Geometry: final body of the model. Coordinates: model frame, mm. A direction names the side the tool comes from. Give positions to 0.01 mm unless a question says otherwise; leave off trailing zeros. Write each loop counter-clockwise with the first axis right and the second up, starting at its lowest first coordinate (ties: lowest second). Pieces come first, ordered by that corner, then holes. Notation, with made-up numbers: M 40,32.5 L 47,32.5 A12 cw 47,48.5 Z; hole C 77,57 d8. An arc over 180 degrees is marked long. Use one line per item in the form item = value. Start each with the question number.
Item 1: Section query B-B on x = -7.5. Return loops of the section in (y, z) (3 decimals), then the cut area to 4 significant figures.
Item 2: Access query for faces 1 (the flat face through (27, 2, 5)), 2 (the flat face through (-27, 2, 15)), 3 (the flat face through (-25.85, 2, -18)). Directions: +Z, -Z, +X, -X, +Y, -Y. A direction counts if a zero-diameter tool reaches every point of the face in a straight line with its end or side. Return the directions, or none.
Item 3: Section query A-A on z = 17. Return loops of the section in (x, y) (3 decimals).
Item 4: Section query C-C on y = 2.4. Give the number of separate pieces and of enclosed holes in the cut face, then the cut area to 3 significant figures.
Item 5: Material intervals for line 1 along Z through (x, y) = (3, 1.9) (3 decimals); line 2 along X through (y, z) = (3.2, 1) (3 decimals); line 3 along X through (y, z) = (1, 24.3) (3 decimals), sorted ascending. Write a range as from..to.
Item 6: Section query D-D on z = -24.3. Return loops of the section in (x, y) (3 decimals), then the cut area to 3 significant figures.
Item 7: Contact query for flat-ended pins moving along their axis: P1, Ø1.5, axis at x = 27.5, y = 2.5, coming from the +Z side; P2, Ø2.5, axis at y = 1.5, z = 18.5, coming from the +X side; P3, Ø1, axis at x = 23, y = 2, coming from the +Z side. Output: stop coordinate, or through.
Item 8: Pull-direction query (X, two-part tool) for faces 4 (the flat face through (28.85, 2, 10)), 5 (the flat face through (-12, 5, 0)), 6 (the cylindrical face through (4.205, 2.465, -22.683)); classes: released by +X, released by -X, zero draft, split by the parting line, or undercut.
from build123d import *

# Parameters (mm, degrees)
SKETCH_1_R      = 1.75
SKETCH_1_W      = 20.75
SKETCH_1_H      = 41.25
EXTRUDE_1_DEPTH = 5
FILLET_1_R      = 8


with BuildPart() as part:
    # 草图1 → 凸台-拉伸1 (new body)
    with BuildSketch(Plane(origin=(0, 0, 0), x_dir=(1, 0, 0), z_dir=(0, 1, 0))):
        Polygon((25.85, -30), (-25.85, -30), (-25.85, -15), (-28.85, -15), (-28.85, -5), (-25.85, -5), (-25.85, 5), (-28.85, 5), (-28.85, 15), (-25.85, 15), (-25.85, 30), (25.85, 30), (25.85, 15), (28.85, 15), (28.85, 5), (25.85, 5), (25.85, -5), (28.85, -5), (28.85, -15), (25.85, -15), align=None)
        with Locations(Location((-4.875, -24.3, 0), (0, 0, 270))):
            Circle(SKETCH_1_R, mode=Mode.SUBTRACT)
        with Locations(Location((4.875, -24.3, 0), (0, 0, 90))):
            Circle(SKETCH_1_R, mode=Mode.SUBTRACT)
        with Locations(Location((4.875, 24.3, 0), (0, 0, 270))):
            Circle(SKETCH_1_R, mode=Mode.SUBTRACT)
        with Locations(Location((-4.875, 24.3, 0), (0, 0, 90))):
            Circle(SKETCH_1_R, mode=Mode.SUBTRACT)
        Rectangle(SKETCH_1_W, SKETCH_1_H, mode=Mode.SUBTRACT)
    extrude(amount=EXTRUDE_1_DEPTH)

    # 圆角1
    fillet_1_edges = [part.edges().sort_by_distance(p)[0] for p in [
        (-25.85, 2.5, -30),
        (25.85, 2.5, -30),
        (25.85, 2.5, 30),
        (-25.85, 2.5, 30),
    ]]
    fillet(fillet_1_edges, radius=FILLET_1_R)


solid = part.part
Answer sheet:
q1.outline = M 0,-30 L 5,-30 L 5,-20.625 L 0,-20.625 Z; M 0,20.625 L 5,20.625 L 5,30 L 0,30 Z
q1.area = 93.75 mm2
q2.face_1 = +X, +Y, -Y
q2.face_2 = +Z, -X, +Y, -Y
q2.face_3 = -Z, -X, +Y, -Y
q3.outline = M -25.85,0 L -10.375,0 L -10.375,5 L -25.85,5 Z; M 10.375,0 L 25.85,0 L 25.85,5 L 10.375,5 Z
q4.separate_pieces = 1
q4.enclosed_holes = 5
q4.area = 2,270 mm2
q5.line_1 = -30..-20.625, 20.625..30
q5.line_2 = -25.85..-10.375, 10.375..25.85
q5.line_3 = -25.512..-6.625, -3.125..3.125, 6.625..25.512
q6.outline = M -25.512,0 L -6.625,0 L -6.625,5 L -25.512,5 Z; M -3.125,0 L 3.125,0 L 3.125,5 L -3.125,5 Z; M 6.625,0 L 25.512,0 L 25.512,5 L 6.625,5 Z
q6.area = 220 mm2
q7.P1 = 15
q7.P2 = 25.85
q7.P3 = 28.51
q8.face_4 = released by +X
q8.face_5 = zero draft
q8.face_6 = undercut
